Here's how the part is built. I have some questions about the finished solid (model axes, mm). Coordinates: 2 decimals unless noted, no trailing zeros. Write each loop counter-clockwise with the first axis right and the second up, starting at its lowest first coordinate (ties: lowest second). Pieces come first, ordered by that corner, then holes.
Item 1: I'm going to push flat-ended pins straight in: pin 1 Ø8 at (x, z) = (13.5, 89) entering from -Y; pin 2 Ø6 at (y, z) = (3.5, 477) entering from -X; pin 3 Ø7.5 at (x, z) = (3.5, 199) entering from +Y. Where does each tip first touch, or does it pass through?
Item 2: If we section it at A-A (z = 63): Please give me the cut outline in (x, y), then the cut area to 3 significant figures.
Item 3: If I drill on line 1 (Y direction, x = 0, z = 242); line 2 (Z direction, x = -7.5, y = 16.5); line 3 (Z direction, x = -0.5, y = -2), over which ranges is the centre line in solid material (lowest first)?
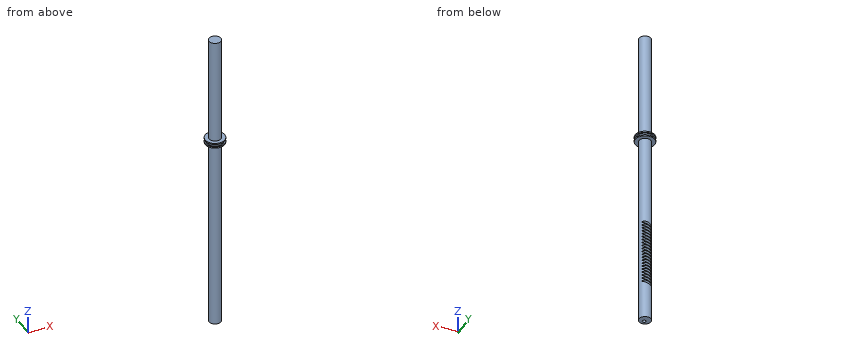
from build123d import *

# Parameters (mm, degrees)
IZIM5_R                     = 11.5
Y_KSEKLIK_EKSTR_ZYON2_DEPTH = 598
IZIM12_R                    = 3.4
KES_EKSTR_ZYON1_DEPTH       = 387


with BuildPart() as part:
    # Çizim5 → Yükseklik-Ekstrüzyon2 (new body)
    with BuildSketch(Plane.XY):
        Circle(IZIM5_R)
    extrude(amount=Y_KSEKLIK_EKSTR_ZYON2_DEPTH)

    # Kes-Süpür2: sweep along a path in Çizim7
    with BuildLine(Plane(origin=(0, 0, 0), x_dir=(1, 0, 0), z_dir=(0, 1, 0))) as kes_s_p_r2_path:
        Line((11.5, -47.002601747), (-17.141789086, -39.043378107))
    # Çizim6 → Kes-Süpür2 (sweep, cut)
    with BuildSketch(Plane(origin=(11.5, 0, 0), x_dir=(0, 0, -1), z_dir=(1, 0, 0))):
        Polygon((-78.362133946, 7), (-80, 11.5), (-81.283711713, 11.5), (-82.921577767, 7), (-84.645319246, 7), (-86.2831853, 11.5), (-87.566897013, 11.5), (-89.204763067, 7), (-90.928504546, 7), (-92.5663706, 11.5), (-93.850082313, 11.5), (-95.487948367, 7), (-97.211689846, 7), (-98.8495559, 11.5), (-100.133267613, 11.5), (-101.771133667, 7), (-103.494875146, 7), (-105.1327412, 11.5), (-106.416452913, 11.5), (-108.054318967, 7), (-109.778060446, 7), (-111.4159265, 11.5), (-112.699638213, 11.5), (-114.337504267, 7), (-116.061245746, 7), (-117.6991118, 11.5), (-118.982823513, 11.5), (-120.620689567, 7), (-122.344431046, 7), (-123.9822971, 11.5), (-125.266008813, 11.5), (-126.903874867, 7), (-128.627616346, 7), (-130.2654824, 11.5), (-131.549194113, 11.5), (-133.187060167, 7), (-134.910801646, 7), (-136.5486677, 11.5), (-137.832379413, 11.5), (-139.470245467, 7), (-141.193986946, 7), (-142.831853, 11.5), (-144.115564713, 11.5), (-145.753430767, 7), (-147.477172246, 7), (-149.1150383, 11.5), (-150.398750013, 11.5), (-152.036616067, 7), (-153.760357546, 7), (-155.3982236, 11.5), (-156.681935313, 11.5), (-158.319801367, 7), (-160.043542846, 7), (-161.6814089, 11.5), (-162.965120613, 11.5), (-164.602986667, 7), (-166.326728146, 7), (-167.9645942, 11.5), (-169.248305913, 11.5), (-170.886171967, 7), (-172.609913446, 7), (-174.2477795, 11.5), (-175.531491213, 11.5), (-177.169357267, 7), (-178.893098746, 7), (-180.5309648, 11.5), (-181.814676513, 11.5), (-183.452542567, 7), (-185.176284046, 7), (-186.8141501, 11.5), (-188.097861813, 11.5), (-189.735727867, 7), (-191.459469346, 7), (-193.0973354, 11.5), (-194.381047113, 11.5), (-196.018913167, 7), (-197.742654646, 7), (-199.3805207, 11.5), (-200.664232413, 11.5), (-202.302098467, 7), (-204.022098467, 7), (-206.232393599, 13.072735964), (-74.431838814, 13.072735964), (-76.642133946, 7), align=None)
    sweep(path=kes_s_p_r2_path.line, mode=Mode.SUBTRACT)

    # Çizim11 → Döndür1 (revolve)
    with BuildSketch(Plane(origin=(0, 0, 0), x_dir=(0, 0, -1), z_dir=(1, 0, 0)), mode=Mode.PRIVATE) as d_nd_r1_sk:
        Polygon((-380, 19), (-380, 11.5), (-390, 11.5), (-390, 19), (-387.5, 19), (-387.5, 16.5), (-382.5, 16.5), (-382.5, 19), align=None)
    revolve(d_nd_r1_sk.sketch.rotate(Axis((0, 0, 0), (0, 0, 1)), 90), axis=Axis((0, 0, 0), (0, 0, 1)))

    # Çizim12 → Kes-Ekstrüzyon1 (cut)
    with BuildSketch(Plane(origin=(0, 0, 0), x_dir=(-1, 0, 0), z_dir=(0, 0, -1))):
        with Locations((0, -3.4)):
            Circle(IZIM12_R)
    extrude(amount=-KES_EKSTR_ZYON1_DEPTH, mode=Mode.SUBTRACT)


solid = part.part
Answer list:
1. pin 1: stops at y = -6.48
1. pin 2: stops at x = -11.49
1. pin 3: stops at y = 11.5
2. outline: circle Ø23 at (0, 0); hole circle Ø6.8 at (0, -3.4)
2. area: 379 mm2
3. line 1: y = -11.5 to -6.8, 0 to 11.5
3. line 2: z = 380 to 382.5, 387.5 to 390
3. line 3: z = 387 to 598
